Geometry: final body of the model. Coordinates: model frame, mm. Face numbers are marked on the shaded views. Give positions to 0.01 mm unless a question says otherwise; leave off trailing zeros. Order: outer loops, then holes, each group sorted by start corner. A loop starts at its lowest first (then second) coordinate and runs counter-clockwise, first axis right, second up. Notation, with made-up numbers: (-35, 25.25) - (-14, 25.25) arc R35 ccw to (-14, 59.25) - close; hole circle Ø10 at (-14.5, -8). An arc over 180 degrees is marked (long way). Put each result on its own line as item: value. Start each with the question number.
1. Mould query, pull axis Y, two halves, no side actions, for the marked faces 1, 2 and 3. Classes: pulls with the +Y half, pulls with the -Y half, needs draft (parallel to the pull), parting line crosses it, or undercut.
2. Section A-A on z = 1.25. Return the cut outline in (x, y), plus the area to 3 significant figures.
3. First-contact query: P1, Ø10, axis at x = -9.5, y = -9, coming from the +Z side; P2, Ø1.5, axis at x = 3, z = 6.5, coming from the -Y side; P3, Ø1.6, axis at x = 21, z = 2, coming from the +Y side; P4, Ø12, axis at x = -26, y = -22, coming from the -Z side. Flat tips, straight axial feed; report the tip coordinate or a pass-through.
4. Ray query, line 1 along X through (y, z) = (-23, 4.25); line 2 along Y through (x, z) = (-13.5, 4.25); line 3 along X through (y, z) = (-18.5, 3.5). Return the intervals inside material, ascending. Write a range as from..to.
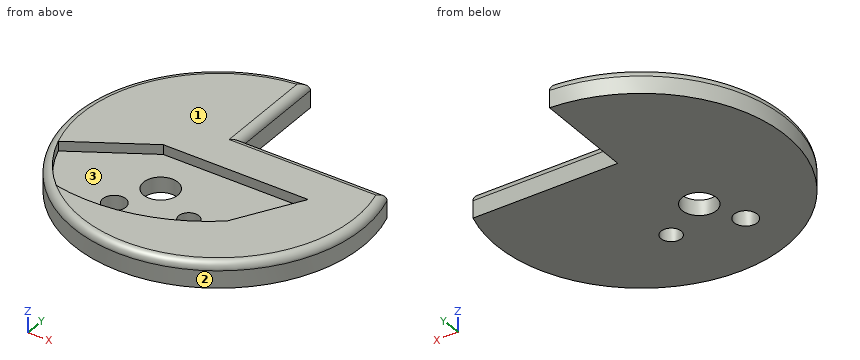
from build123d import *

# Parameters (mm, degrees)
F1_DEPTH = 7.874
F2_R     = 2.452841
F4_DEPTH = 3.048
F5_R     = 5.404397
F5_R_2   = 3.62081
F5_R_3   = 3.18203
F6_DEPTH = 25.4


with BuildPart() as f1:
    # F0 (on Top) → F1 (new body)
    with BuildSketch(Plane.XY):
        with BuildLine():
            Line((-2.126512, 14.08814), (-2.126512, 45.570451))
            ThreePointArc((-2.126512, 45.570451), (-25.951063, -37.519734), (43.390234, 14.08814))
            Line((43.390234, 14.08814), (-2.126512, 14.08814))
        make_face()
    extrude(amount=F1_DEPTH)

    # F2
    f2_edges = [f1.edges().sort_by_distance(p)[0] for p in [
        (20.631861, 14.08814, 7.874),
        (-2.126512, 29.829296, 7.874),
        (-25.951063, -37.519734, 7.874),
    ]]
    fillet(f2_edges, radius=F2_R)

    # F3 (on face) → F4 (cut)
    with BuildSketch(Plane.XY.offset(7.874)):
        with BuildLine():
            ThreePointArc((-40.823762, -14.029525), (-36.271678, -23.40454), (-29.605426, -31.415376))
            ThreePointArc((-29.605426, -31.415376), (-5.306065, -31.015874), (16.444359, -20.174399))
            Line((16.444359, -20.174399), (28.192235, 0))
            Line((28.192235, 0), (-17.349953, 0))
            Line((-17.349953, 0), (-40.823762, -14.029525))
        make_face()
    extrude(amount=-F4_DEPTH, mode=Mode.SUBTRACT)

    # F5 (on face) → F6 (cut)
    with BuildSketch(Plane.XY.offset(4.826)):
        with Locations((-8.902777, -13.591718)):
            Circle(F5_R)
        with Locations((-15.087833, -25.941195)):
            Circle(F5_R_2)
        with Locations((5.261666, -21.411046)):
            Circle(F5_R_3)
    extrude(amount=-F6_DEPTH, mode=Mode.SUBTRACT)


solid = f1.part
Resolved:
1. face 1: needs draft
1. face 2: parting line crosses it
1. face 3: undercut
2. outline: (-2.13, 14.09) - (-2.13, 45.57) arc R45.62 ccw (long way) to (43.39, 14.09) - close; hole circle Ø7.24 at (-15.09, -25.94); hole circle Ø10.81 at (-8.9, -13.59); hole circle Ø6.36 at (5.26, -21.41)
2. area: 5,300 mm^2
3. P1: z = 4.83
3. P2: y = -45.51
3. P3: y = 14.09
3. P4: z = 0
4. line 1: -39.4..-17.2, -12.98..2.5, 8.02..39.4
4. line 2: -43.58..-29.2, -22.69..-16.43, -10.75..43.58
4. line 3: -41.7..-11.16, -6.64..3.98, 6.55..41.7
